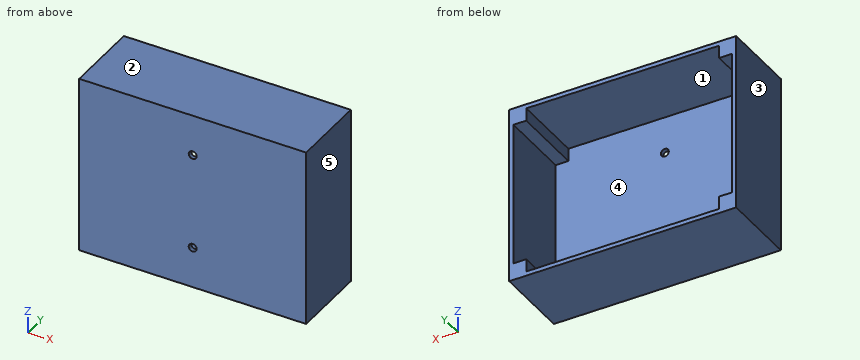
Autodesk Inventor part; units mm, degrees
ref_plane "YZ Plane" through (0, 0, 0) normal (1, 0, 0) x (0, 1, 0)
ref_plane "XZ Plane" through (0, 0, 0) normal (0, 1, 0) x (-1, 0, 0)
ref_plane "XY Plane" through (0, 0, 0) normal (0, 0, 1) x (1, 0, 0)
sketch "Sketch1" plane through (0, 0, 0) normal (0, 1, 0) x (-1, 0, 0)
  line L0 (-59.7535, -47.0027) -> (59.7535, -47.0027)
  line L1 (59.7535, -47.0027) -> (59.7535, 47.0027)
  line L2 (59.7535, 47.0027) -> (-59.7535, 47.0027)
  line L3 (-59.7535, 47.0027) -> (-59.7535, -47.0027)
  line L4 (-59.7535, -47.0027) -> (59.7535, 47.0027) construction
  line L5 (59.7535, -47.0027) -> (-59.7535, 47.0027) construction
  point P0 (0, 0)
  dimension "d0" = 119.507
  dimension "d1" = 94.0054
extrude "Extrusion1" add sketch "Sketch1" along normal mid plane 2.2606
sketch "Sketch2" plane through (0, 1.1303, 0) normal (0, 1, 0) x (1, 0, 0)
  line L0 (-59.7535, 47.0027) -> (-59.7535, -47.0027)
  line L1 (59.7535, -47.0027) -> (59.7535, 47.0027)
  line L2 (-59.7535, -47.0027) -> (59.7535, -47.0027)
  line L3 (59.7535, -47.0027) -> (59.7535, 47.0027)
  line L4 (59.7535, 47.0027) -> (-59.7535, 47.0027)
  line L5 (-59.7535, 47.0027) -> (-59.7535, -47.0027)
  line L6 (57.4929, -44.7421) -> (-57.4929, 44.7421) construction
  line L7 (-57.4929, -44.7421) -> (57.4929, 44.7421) construction
  line L8 (-59.7535, -47.0027) -> (59.7535, -47.0027)
  line L9 (-59.7535, -47.0027) -> (-50.7619, -47.0027)
  line L10 (-59.7535, -38.0111) -> (-59.7535, -47.0027)
  line L11 (-59.7535, 47.0027) -> (-50.7619, 47.0027)
  line L12 (-59.7535, 38.0111) -> (-59.7535, 47.0027)
  line L13 (59.7535, 47.0027) -> (-59.7535, 47.0027)
  line L14 (59.7535, 47.0027) -> (50.7619, 47.0027)
  line L15 (59.7535, 38.0111) -> (59.7535, 47.0027)
  line L16 (59.7535, -47.0027) -> (50.7619, -47.0027)
  line L17 (59.7535, -38.0111) -> (59.7535, -47.0027)
  line L18 (-50.7619, -44.7421) -> (-50.7619, -38.0111)
  line L19 (-50.7619, -38.0111) -> (-57.4929, -38.0111)
  line L20 (-57.4929, 38.0111) -> (-50.7619, 38.0111)
  line L21 (-50.7619, 38.0111) -> (-50.7619, 44.7421)
  line L22 (50.7619, 38.0111) -> (57.4929, 38.0111)
  line L23 (50.7619, 44.7421) -> (50.7619, 38.0111)
  line L24 (57.4929, -38.0111) -> (50.7619, -38.0111)
  line L25 (50.7619, -38.0111) -> (50.7619, -44.7421)
  line L26 (-50.7619, -44.7421) -> (50.7619, -44.7421)
  line L27 (57.4929, -38.0111) -> (57.4929, 38.0111)
  line L28 (50.7619, 44.7421) -> (-50.7619, 44.7421)
  line L29 (-57.4929, 38.0111) -> (-57.4929, -38.0111)
  point P0 (0, 0)
  dimension "d4" = 114.9858
  dimension "d5" = 89.4842
  dimension "d6" = 8.9916
  dimension "d7" = 8.9916
  dimension "d10" = 8.9916
  dimension "d11" = 8.9916
extrude "Extrusion2" add sketch "Sketch2" along normal blind 38.1
sketch "Sketch3" plane through (0, 1.1303, 0) normal (0, 1, 0) x (1, 0, 0)
  circle A0 centre (0, -25.4) radius 2.0828
  circle A1 centre (0, 25.4) radius 2.0828
  point P0 (0, 0)
  dimension "d18" = 4.1656
  dimension "d19" = 4.1656
extrude "Extrusion3" cut sketch "Sketch3" against normal through all
properties part number "546-1590BBS-4.7x3.7-Enclosure"
CAD build for the part. Positions are in the model's coordinates, mm. Face numbers are marked on the shaded views. A direction names the side the tool comes from. Coordinates: 2 decimals unless noted, no trailing zeros. Write each loop counter-clockwise with the first axis right and the second up, starting at its lowest first coordinate (ties: lowest second). Pieces come first, ordered by that corner, then holes. Notation, with made-up numbers: (44.5, 11.25) -> (57.5, 11.25) arc R13 cw to (57.5, 25.25) -> close; hole circle Ø8 at (-14.75, 5.5). An arc over 180 degrees is marked (long way). Return JSON: item names as keys, results as strings. Group by question number.
Q1. Cut at D-D, the plane z = 16. Give the cut face in (x, y).
Q2. Drill centre lines: line 1 (Z direction, x = 0, y = 0); line 2 (Z direction, x = -23, y = 14.5); line 3 (X direction, y = 13, z = -23). Where is each one in solid material? Low to high.
Q3. Cut at B-B, the plane x = 0. Give the cut face in (y, z), then the cut area to 3 significant figures.
Q4. Cut at A-A, the plane z = -25.4. Give the cut face in (x, y), then the cut area to 3 significant figures.
Q5. Flat gauge pins, fed straight in: pin 1 (3.5 mm diameter, centred on x = 0, z = -25.4, fed in from -Y); pin 2 (1.5 mm diameter, centred on x = 37, z = -8, fed in from +Y). Where does each tip first touch, or does it go through?
Q6. Which spindle directions (+Z, -Z, +X, -X, +Y, -Y) get a long thin tool onto all of the face, cutting with end or side? Do the marked faces 1 and 2. Say none if no direction does.
Q7. Pull direction X, two halves, no side cores. Call the marked faces 3, 4 and 5: released by +X, released by -X, zero draft, split by the parting line, or undercut.
Q8. Cut at C-C, the plane y = 12.5. Give the cut face in (x, z), then the cut area to 3 significant figures.
Returned:
{
 "1": {"outline": "(-59.75, -1.13) -> (59.75, -1.13) -> (59.75, 39.23) -> (57.49, 39.23) -> (57.49, 1.13) -> (-57.49, 1.13) -> (-57.49, 39.23) -> (-59.75, 39.23) -> close"},
 "2": {"line 1": "z = -47 to -27.48, -23.32 to 23.32, 27.48 to 47", "line 2": "z = -47 to -44.74, 44.74 to 47", "line 3": "x = -59.75 to -57.49, 57.49 to 59.75"},
 "3": {"outline": "(-1.13, -47) -> (39.23, -47) -> (39.23, -44.74) -> (1.13, -44.74) -> (1.13, -27.48) -> (-1.13, -27.48) -> close; (-1.13, -23.32) -> (1.13, -23.32) -> (1.13, 23.32) -> (-1.13, 23.32) -> close; (-1.13, 27.48) -> (1.13, 27.48) -> (1.13, 44.74) -> (39.23, 44.74) -> (39.23, 47) -> (-1.13, 47) -> close", "area": "366 mm2"},
 "4": {"outline": "(-59.75, -1.13) -> (-2.08, -1.13) -> (-2.08, 1.13) -> (-57.49, 1.13) -> (-57.49, 39.23) -> (-59.75, 39.23) -> close; (2.08, -1.13) -> (59.75, -1.13) -> (59.75, 39.23) -> (57.49, 39.23) -> (57.49, 1.13) -> (2.08, 1.13) -> close", "area": "433 mm2"},
 "5": {"pin 1": "passes through", "pin 2": "stops at y = 1.13"},
 "6": {"face 1": "+Y", "face 2": "+Z, +X, -X, +Y, -Y"},
 "7": {"face 3": "released by -X", "face 4": "undercut", "face 5": "released by +X"},
 "8": {"outline": "(-59.75, -47) -> (59.75, -47) -> (59.75, 47) -> (-59.75, 47) -> close; hole (-57.49, -38.01) -> (-50.76, -38.01) -> (-50.76, -44.74) -> (50.76, -44.74) -> (50.76, -38.01) -> (57.49, -38.01) -> (57.49, 38.01) -> (50.76, 38.01) -> (50.76, 44.74) -> (-50.76, 44.74) -> (-50.76, 38.01) -> (-57.49, 38.01) -> close", "area": "1,130 mm2"}
}
